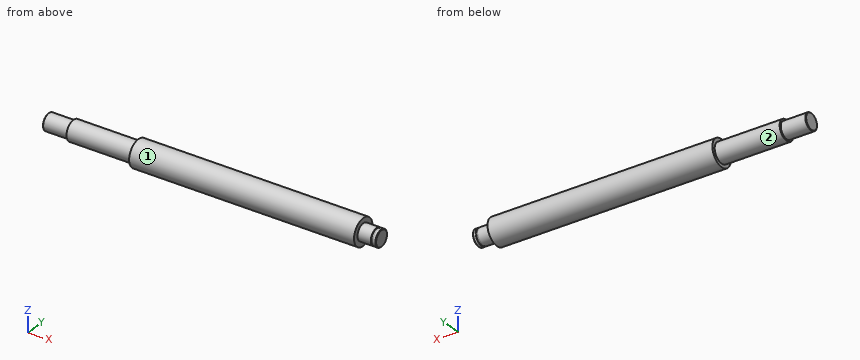
from build123d import *

# Parameters (mm, degrees)
SKETCH_2_W     = 1.15
SKETCH_2_H     = 0.4
CHAMFER_1_SIZE = 0.3


with BuildPart() as part:
    # Sketch 1 → Revolve 1 (revolve)
    with BuildSketch(Plane.XY, mode=Mode.PRIVATE) as revolve_1_sk:
        Polygon((-100, 0), (100, 0), (100, 5), (89, 5), (89, 8), (-46, 8), (-46, 6), (-85, 6), (-85, 5), (-100, 5), align=None)
    revolve(revolve_1_sk.sketch.rotate(Axis((-100, 0, 0), (1, 0, 0)), 90), axis=Axis((-100, 0, 0), (1, 0, 0)))

    # Sketch 2 → Cut-Revolve 1 (revolve, cut)
    with BuildSketch(Plane.XY, mode=Mode.PRIVATE) as cut_revolve_1_sk:
        with Locations((97.575, 4.8)):
            Rectangle(SKETCH_2_W, SKETCH_2_H)
    revolve(cut_revolve_1_sk.sketch.rotate(Axis((89, 0, 0), (1, 0, 0)), 90), axis=Axis((89, 0, 0), (1, 0, 0)), mode=Mode.SUBTRACT)

    # Chamfer 1
    chamfer_1_edges = [part.edges().sort_by_distance(p)[0] for p in [
        (-100, 0, -5),
        (100, 0, -5),
    ]]
    chamfer(chamfer_1_edges, length=CHAMFER_1_SIZE)


solid = part.part
Could you check a few things on this model? Use its own coordinates, in mm. Face numbers are marked on the shaded views. A direction names the side the tool comes from. Round coordinates to 2 decimals unless told otherwise and drop trailing zeros. Write each loop counter-clockwise with the first axis right and the second up, starting at its lowest first coordinate (ties: lowest second). Pieces come first, ordered by that corner, then holes. Notation, with made-up numbers: (12, 30) - (62, 30) arc R17 cw to (62, 63) - close; hole circle Ø8 at (26, 38). An arc over 180 degrees is marked (long way). Put each result on its own line as item: value. Start each with the question number.
(1) I want a section at A-A, the plane y = 0. Please give me the cut outline in (x, z).
(2) Will these pins go through, and if not, where does the flat tip stop? pin 1 (1.5 mm diameter, centred on x = -43.5, z = -3, fed in from +Y); pin 2 (2 mm diameter, centred on x = 34.5, z = 2, fed in from +Y); pin 3 (3 mm diameter, centred on x = -80, y = -6.5, fed in from +Z).
(3) I want a section at C-C, the plane x = -53. Please give me the cut outline in (y, z).
(4) I need wall thicknesses on probe 1 along Z at (x, y) = (86.5, -0.25); probe 2 along Y at (x, z) = (-83, 0); probe 3 along Y at (x, z) = (27.5, 6.25). Which ranges of each line are inside material? Lowest first, please.
(5) For the marked faces 1 and 2, which set-ups out of +Z, -Z, +X, -X, +Y, -Y let a thin tool reach every point of the face, with its end or its side?
(6) I want a section at D-D, the plane x = 24.5. Please give me the cut outline in (y, z), plus the area to 3 significant figures.
Here are the results:
1. outline: (-100, -4.7) - (-99.7, -5) - (-85, -5) - (-85, -6) - (-46, -6) - (-46, -8) - (89, -8) - (89, -5) - (97, -5) - (97, -4.6) - (98.15, -4.6) - (98.15, -5) - (99.7, -5) - (100, -4.7) - (100, 4.7) - (99.7, 5) - (98.15, 5) - (98.15, 4.6) - (97, 4.6) - (97, 5) - (89, 5) - (89, 8) - (-46, 8) - (-46, 6) - (-85, 6) - (-85, 5) - (-99.7, 5) - (-100, 4.7) - close
2. pin 1: stops at y = 7.68
2. pin 2: stops at y = 7.94
2. pin 3: stops at z = 3.32
3. outline: circle Ø12 at (0, 0)
4. probe 1: z = -8 to 8
4. probe 2: y = -6 to 6
4. probe 3: y = -4.99 to 4.99
5. face 1: +X, -X
5. face 2: -X
6. outline: circle Ø16 at (0, 0)
6. area: 201 mm^2
